```python
from build123d import *

# Parameters (mm, degrees)
SKETCH1_W                  = 38.1
SKETCH1_H                  = 38.1
BOSS_EXTRUDE1_DEPTH        = 38.1
SKETCH2_W                  = 35.814
SKETCH2_H                  = 35.814
CUT_EXTRUDE1_DEPTH         = 58.15
HOLE1_D                    = 12.7254
HOLE1_DEPTH                = 38.1
M3_5_CLEARANCE_HOLE1_D     = 4.064
M3_5_CLEARANCE_HOLE1_DEPTH = 38.1
M3_CLEARANCE_HOLE1_D       = 3.556
M3_CLEARANCE_HOLE1_DEPTH   = 38.1
HOLE2_D                    = 12.7254
M3_5_CLEARANCE_HOLE2_D     = 4.064
M3_CLEARANCE_HOLE2_D       = 3.556
FILLET1_R                  = 1.27


with BuildPart() as part:
    # Sketch1 → Boss-Extrude1 (new body)
    with BuildSketch(Plane.XZ):
        Rectangle(SKETCH1_W, SKETCH1_H)
    extrude(amount=-BOSS_EXTRUDE1_DEPTH)

    # Sketch2 → Cut-Extrude1 (cut, through all)
    with BuildSketch(Plane.ZY.offset(19.05)):
        with Locations((-1.143, 20.193)):
            Rectangle(SKETCH2_W, SKETCH2_H)
    extrude(amount=-CUT_EXTRUDE1_DEPTH, mode=Mode.SUBTRACT)

    # Hole1
    with Locations(Plane.XY.offset(19.05)):
        with Locations((0, 19.05)):
            Hole(HOLE1_D / 2, depth=HOLE1_DEPTH)

    # M3.5 Clearance Hole1
    with Locations(Plane.XY.offset(19.05)):
        with Locations((-9.525, 19.05), (9.525, 19.05)):
            Hole(M3_5_CLEARANCE_HOLE1_D / 2, depth=M3_5_CLEARANCE_HOLE1_DEPTH)

    # M3 Clearance Hole1
    with Locations(Plane.XY.offset(19.05)):
        with Locations((12.135202787, 12.135202787), (-5.579615818, 32.520384182), (-12.135202787, 25.964797213), (5.579615818, 32.520384182), (12.135202787, 25.964797213), (13.470384182, 32.520384182), (-13.470384182, 5.579615818), (-13.470384182, 32.520384182), (13.470384182, 5.579615818), (6.914797213, 25.964797213), (6.914797213, 12.135202787), (0, 9.271), (-6.914797213, 12.135202787), (-6.914797213, 25.964797213), (0, 28.829), (-12.135202787, 12.135202787), (-5.579615818, 5.579615818), (5.579615818, 5.579615818)):
            Hole(M3_CLEARANCE_HOLE1_D / 2, depth=M3_CLEARANCE_HOLE1_DEPTH)

    # Hole2 (through all)
    with Locations(Plane(origin=(0, 2.286, 0), x_dir=(1, 0, 0), z_dir=(0, 1, 0))):
        with Locations((0, 0)):
            Hole(HOLE2_D / 2)

    # M3.5 Clearance Hole2 (through all)
    with Locations(Plane(origin=(0, 2.286, 0), x_dir=(1, 0, 0), z_dir=(0, 1, 0))):
        with Locations((-9.525, 0), (9.525, 0)):
            Hole(M3_5_CLEARANCE_HOLE2_D / 2)

    # M3 Clearance Hole2 (through all)
    with Locations(Plane(origin=(0, 2.286, 0), x_dir=(1, 0, 0), z_dir=(0, 1, 0))):
        with Locations((5.579615818, -13.470384182), (12.135202787, -6.914797213), (-5.579615818, -13.470384182), (-12.135202787, -6.914797213), (-5.579615818, 13.470384182), (-12.135202787, 6.914797213), (5.579615818, 13.470384182), (12.135202787, 6.914797213), (-13.470384182, 13.470384182), (13.470384182, -13.470384182), (13.470384182, 13.470384182), (-13.470384182, -13.470384182), (-6.914797213, 6.914797213), (-6.914797213, -6.914797213), (0, -9.779), (6.914797213, -6.914797213), (6.914797213, 6.914797213), (0, 9.779)):
            Hole(M3_CLEARANCE_HOLE2_D / 2)

    # Fillet1
    fillet1_edges = [part.edges().sort_by_distance(p)[0] for p in [
        (19.05, 38.1, 17.907),
        (-19.05, 1.143, -19.05),
        (19.05, 1.143, -19.05),
        (-19.05, 38.1, 17.907),
    ]]
    fillet(fillet1_edges, radius=FILLET1_R)


solid = part.part
```
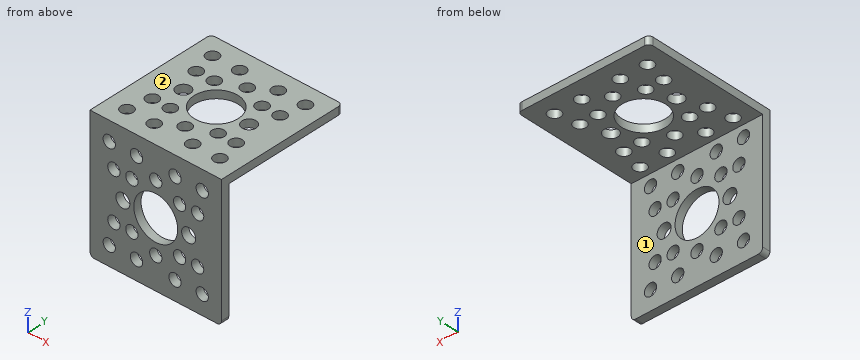
Here's how the part is built. I have some questions about the finished solid (model axes, mm). Face numbers are marked on the shaded views. A direction names the side the tool comes from. Round coordinates to 2 decimals unless told otherwise and drop trailing zeros. Write each loop counter-clockwise with the first axis right and the second up, starting at its lowest first coordinate (ties: lowest second). Pieces come first, ordered by that corner, then holes. Notation, with made-up numbers: M 23.5,-20 L 67.5,-20 A14 ccw 67.5,-4 Z; hole C 29,51 d4. An arc over 180 degrees is marked long. Answer as CSV lines item,"result". Start each with the question number.
1. Suppose I cut it at B-B on z = 0. Write out the boundary of the cut face in (x, y), then the cut area to 3 significant figures.
2. Suppose I cut it at D-D on y = 30. Write out the boundary of the cut face in (x, z), then the cut area to 3 significant figures.
3. Suppose I cut it at A-A on x = 0. Count the separate pieces of the cut face and the enclosed holes in it, then the cut area to 3 significant figures.
4. I need wall thicknesses on probe 1 along Y at (x, z) = (0, 17.5); probe 2 along Y at (x, z) = (-13, 17.5); probe 3 along Z at (x, y) = (-4.5, 8). Which ranges of each line are inside material? Lowest first, please.
5. Suppose I cut it at C-C on y = 19.05. Write out the boundary of the cut face in (x, z), then the cut area to 3 significant figures.
6. I'm going to push flat-ended pins straight in: pin 1 Ø5.5 at (x, z) = (6.91, -6.91) entering from +Y; pin 2 Ø4 at (x, y) = (0, 9.271) entering from -Z. Where does each tip first touch, or does it pass through?
7. On a 3-axis mill with a long thin cutter (end or side, diameter ignored), from which of +Z, -Z, +X, -X, +Y, -Y can I reach the whole of each face in a straight line? I mean the marked faces 1 and 2. Say none if no direction works.
Check result:
1,outline,"M -19.05,0 L -11.56,0 L -11.56,2.29 L -19.05,2.29 Z; M -7.49,0 L -6.36,0 L -6.36,2.29 L -7.49,2.29 Z; M 6.36,0 L 7.49,0 L 7.49,2.29 L 6.36,2.29 Z; M 11.56,0 L 19.05,0 L 19.05,2.29 L 11.56,2.29 Z"
1,area,"39.4 mm2"
2,outline,"M -19.05,16.76 L -1.34,16.76 L -1.34,19.05 L -19.05,19.05 Z; M 1.34,16.76 L 19.05,16.76 L 19.05,19.05 L 1.34,19.05 Z"
2,area,"81.0 mm2"
3,separate pieces,"7"
3,enclosed holes,"0"
3,area,"78.3 mm2"
4,probe 1,"y = 0 to 7.49, 11.05 to 12.69, 25.41 to 27.05, 30.61 to 38.1"
4,probe 2,"y = 0 to 3.86, 7.29 to 10.58, 13.69 to 24.41, 27.52 to 30.81, 34.24 to 38.1"
4,probe 3,"z = 16.76 to 19.05"
5,outline,"M -19.05,16.76 L -11.56,16.76 L -11.56,19.05 L -19.05,19.05 Z; M -7.49,16.76 L -6.36,16.76 L -6.36,19.05 L -7.49,19.05 Z; M 6.36,16.76 L 7.49,16.76 L 7.49,19.05 L 6.36,19.05 Z; M 11.56,16.76 L 19.05,16.76 L 19.05,19.05 L 11.56,19.05 Z"
5,area,"39.4 mm2"
6,pin 1,"stops at y = 2.29"
6,pin 2,"stops at z = 16.76"
7,face 1,"-Z, +X, -X, +Y"
7,face 2,"+Z, +X, -X, +Y, -Y"
